Answer from the drawing. Dimensions are ordinates in mm from the lowest x, y and z of the part. Round coordinates to 2 decimals unless told otherwise and drop trailing zeros. Write each loop counter-clockwise with the first axis right and the second up, starting at its lowest first coordinate (ties: lowest second). Pieces come first, ordered by that corner, then holes. Notation, with made-up numbers: (23.25, -25) -> (52.25, -25) arc R13 cw to (52.25, -13) -> close; hole circle Ø10 at (50, -2). An arc over 180 degrees is marked (long way). Return JSON: item names as keys, results as strings. Group by question number.
(1) A cutting plane is placed at A-A on x = 6.5. Give the vertices of the cut face in (y, z), then the cut area to 3 significant figures.
(2) A cutting plane is placed at D-D on x = 38. Give the vertices of the cut face in (y, z).
(3) Given pin 1 (1 mm diameter, centred on x = 54.5, y = 6, fed in from -Z), flat-ended and moving along its own axis, determine where the tip first touches the part or whether it passes through.
(4) Straight lines are drawn through the part: line 1 (X direction, y = 3.5, z = 0.55); line 2 (Y direction, x = 58.5, z = 1.5); line 3 (Y direction, x = 27, z = 0.95). For each, find the intervals that lie inside material, in ascending order.
(5) A cutting plane is placed at C-C on y = 4.25. Give the vertices of the cut face in (x, z).
(6) A cutting plane is placed at B-B on z = 1.4. Give the vertices of the cut face in (x, y), then the cut area to 3 significant figures.
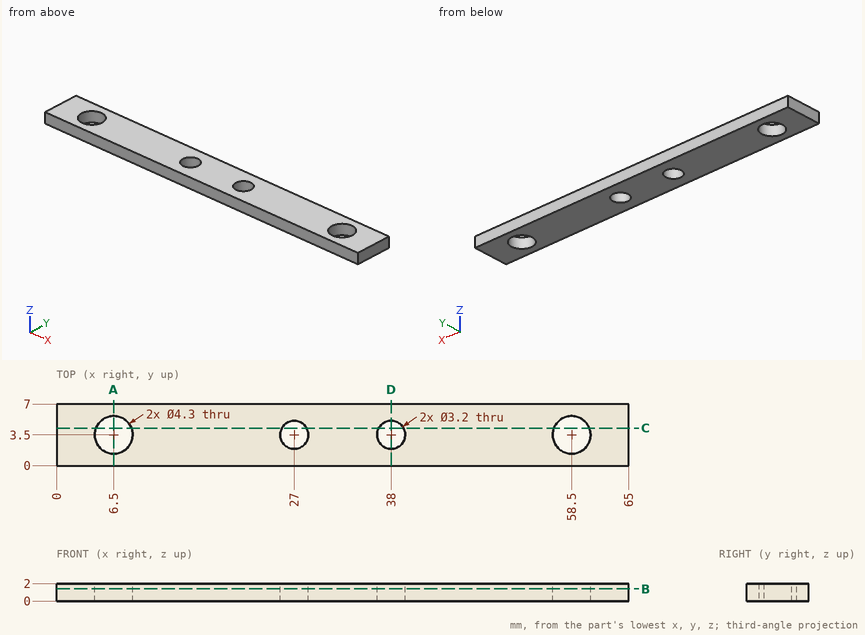
Checks:
{
 "1": {"outline": "(0, 0) -> (1.35, 0) -> (1.35, 2) -> (0, 2) -> close; (5.65, 0) -> (7, 0) -> (7, 2) -> (5.65, 2) -> close", "area": "5.40 mm^2"},
 "2": {"outline": "(0, 0) -> (1.9, 0) -> (1.9, 2) -> (0, 2) -> close; (5.1, 0) -> (7, 0) -> (7, 2) -> (5.1, 2) -> close"},
 "3": {"pin 1": "stops at z = 0"},
 "4": {"line 1": "x = 0 to 4.35, 8.65 to 25.4, 28.6 to 36.4, 39.6 to 56.35, 60.65 to 65", "line 2": "y = 0 to 1.35, 5.65 to 7", "line 3": "y = 0 to 1.9, 5.1 to 7"},
 "5": {"outline": "(0, 0) -> (4.49, 0) -> (4.49, 2) -> (0, 2) -> close; (8.51, 0) -> (25.59, 0) -> (25.59, 2) -> (8.51, 2) -> close; (28.41, 0) -> (36.59, 0) -> (36.59, 2) -> (28.41, 2) -> close; (39.41, 0) -> (56.49, 0) -> (56.49, 2) -> (39.41, 2) -> close; (60.51, 0) -> (65, 0) -> (65, 2) -> (60.51, 2) -> close"},
 "6": {"outline": "(0, 0) -> (65, 0) -> (65, 7) -> (0, 7) -> close; hole circle Ø4.3 at (6.5, 3.5); hole circle Ø3.2 at (27, 3.5); hole circle Ø3.2 at (38, 3.5); hole circle Ø4.3 at (58.5, 3.5)", "area": "410 mm^2"}
}
